Here's the drawing with two shaded views (mm, measured from the low corner). I have some questions. Round coordinates to 2 decimals unless told otherwise and drop trailing zeros. Loops run counter-clockwise (first coordinate to the right, second up) from the corner with the lowest first, then second, coordinate; pieces in that order, holes last.
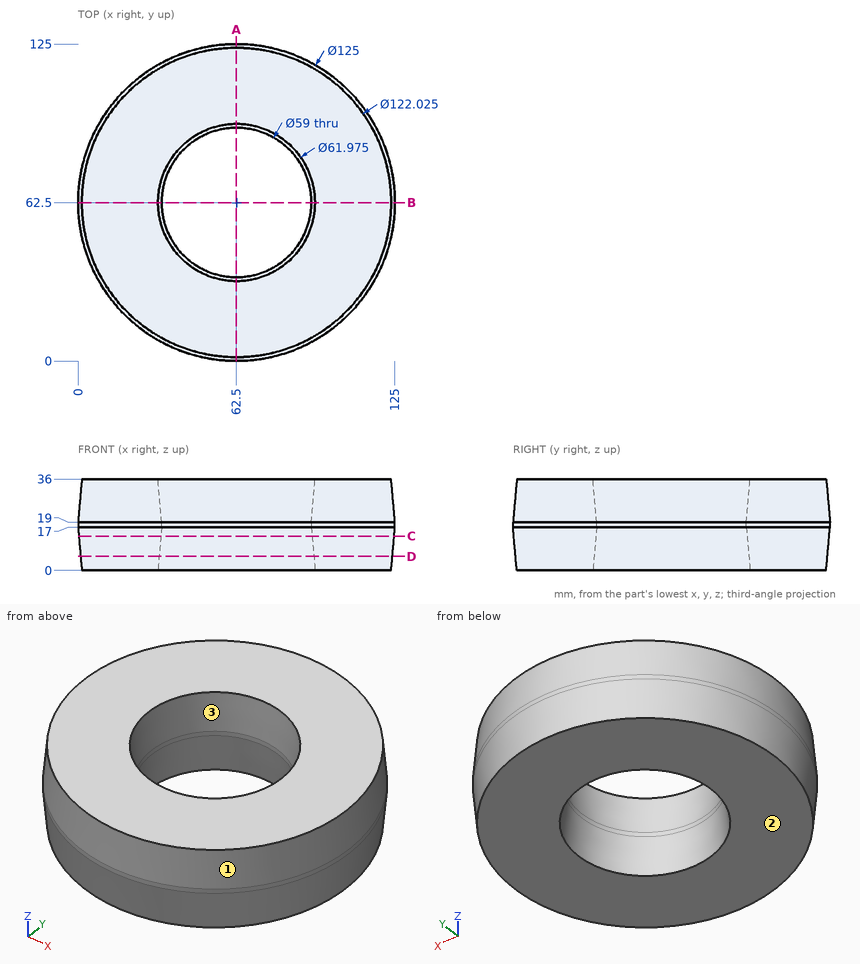
Item 1: If we section it at D-D, the plane z = 5.5: Please give me the cut outline in (x, y), then the cut area to 3 significant figures.
Results list:
outline: circle Ø122.99 at (62.5, 62.5); hole circle Ø61.01 at (62.5, 62.5)
area: 8,960 mm2
Item 2: If we section it at C-C, the plane z = 13.5: Please give me the cut outline in (x, y).
Results list:
outline: circle Ø124.39 at (62.5, 62.5); hole circle Ø59.61 at (62.5, 62.5)
Item 3: If we section it at A-A, the plane x = 62.5: Please give me the cut outline in (y, z), then the cut area to 4 significant figures.
Results list:
outline: (0, 17) - (1.49, 0) - (31.51, 0) - (33, 17) - (33, 19) - (31.51, 36) - (1.49, 36) - (0, 19) - close; (92, 17) - (93.49, 0) - (123.51, 0) - (125, 17) - (125, 19) - (123.51, 36) - (93.49, 36) - (92, 19) - close
area: 2,275 mm2
Item 4: If I drill on line 1 along X through (y, z) = (62, 17) (1 decimal); line 2 along Y through (x, z) = (67, 24), over which ranges is the centre line in solid material (lowest first)?
Results list:
line 1: x = 0 to 33, 92 to 125
line 2: y = 0.6 to 32.9, 92.1 to 124.4
Item 5: Will these pins go through, and if not, where does the flat tip stop? pin 1 (1 mm diameter, centred on x = 79, z = 28, fed in from +Y); pin 2 (2 mm diameter, centred on y = 81.5, z = 20.5, fed in from -X); pin 3 (8 mm diameter, centred on x = 23.5, z = 4.5, fed in from +Y); pin 4 (3 mm diameter, centred on x = 23.5, y = 79, fed in from -Z).
Results list:
pin 1: stops at y = 122.11
pin 2: stops at x = 2.77
pin 3: stops at y = 112.99
pin 4: stops at z = 0
Item 6: We'd pull the mould along Y, two halves only. Please class the marked faces 1, 2 and 3: released by +Y, released by -Y, zero draft, split by the parting line, or undercut.
Results list:
face 1: split by the parting line
face 2: zero draft
face 3: undercut
